The listing builds one solid part. Answer for the finished solid, in the listing's coordinates (mm). A direction names the side the tool comes from. Give positions to 0.01 mm unless a question says otherwise; leave off trailing zeros. Order: outer loops, then holes, each group sorted by start corner. A loop starts at its lowest first (then second) coordinate and runs counter-clockwise, first axis right, second up. Notation, with made-up numbers: (-32.5, 87.5) - (9.5, 87.5) arc R17 ccw to (9.5, 100.5) - close; hole circle Ø3 at (52, 78.5). An arc over 180 degrees is marked (long way). Use CSV: the item, a comma, the result in double quotes.
```python
from build123d import *

# Parameters (mm, degrees)
F0_R            = 100
F1_DEPTH        = 22
F2_R            = 3
F3_DEPTH        = 160
F3_COPIES_COUNT = 8
F4_R            = 15
F5_DEPTH        = 23
F6_R            = 5
F7_DEPTH        = 150


# Not quite as in the source:
# - a pattern or mirror of a feature is missing from the dataset's text; its kind, count and spacing are read off the source's solid


with BuildPart() as f1:
    # F0 (on Top) → F1 (new body)
    with BuildSketch(Plane.XY):
        Circle(F0_R)
    extrude(amount=F1_DEPTH)

    # F2 (on face) → F3 (join)
    with BuildSketch(Plane.XY.offset(22)):
        with Locations((10, 0)):
            Circle(F2_R)
        with Locations((30, 0)):
            Circle(F2_R)
        with Locations((50, 0)):
            Circle(F2_R)
        with Locations((70, 0)):
            Circle(F2_R)
        with Locations((90, 0)):
            Circle(F2_R)
    f3 = extrude(amount=F3_DEPTH)

    # F3_copies: F3 ×8 about axis
    f3_copies_axis = Axis((0, 0, 0), (0, 0, 1))
    for i in range(1, F3_COPIES_COUNT):
        add(f3.rotate(f3_copies_axis, i * 360 / F3_COPIES_COUNT))

    # F4 (on face) → F5 (join)
    with BuildSketch(Plane.XY):
        Circle(F4_R)
    extrude(amount=-F5_DEPTH)

    # F6 (on face) → F7 (join)
    with BuildSketch(Plane(origin=(0, 0, -23), x_dir=(1, 0, 0), z_dir=(0, 0, -1))):
        Circle(F6_R)
    extrude(amount=F7_DEPTH)


solid = f1.part
```
Item 1: The mould has two halves that part along X. Classify faces 3 (the face through (95.38, 30.04, 10.85)), 4 (the face through (-1, 1, 22)), 5 (the face through (-1, -21, 0)): +X half, -X half, draft (parallel to the pull), parting line (faces both ways), or undercut.
Taken from the geometry:
face 3,"parting line"
face 4,"undercut"
face 5,"draft"
Item 2: The part is cut by section B-B (z = -141). Give the vertices of the cut face in (x, y), and give its area (3 significant figures).
Taken from the geometry:
outline,"circle Ø10 at (0, 0)"
area,"78.5 mm^2"
Item 3: Find the intervals of material crossed by line 1 along X through (y, z) = (-63.5, 132); line 2 along Z through (x, y) = (-13, -34); line 3 along X through (y, z) = (-30, 30.5), in increasing order.
Taken from the geometry:
line 1,"-66.64 to -60.64, 60.64 to 66.64"
line 2,"0 to 22"
line 3,"-3 to 3"
Item 4: The part is cut by section A-A (z = 17.5). Give the vertices of the cut face in (x, y).
Taken from the geometry:
outline,"circle Ø200 at (0, 0)"
Item 5: Each of these flat-tipped pins is pushed along its axis until it touches: pin 1 (24 mm diameter, centred on x = 1.5, y = -5.5, fed in from -Z); pin 2 (1.5 mm diameter, centred on x = -29.5, z = 14, fed in from -Y); pin 3 (1 mm diameter, centred on x = 76.5, y = 57, fed in from -Z); pin 4 (1.5 mm diameter, centred on y = 46, z = 39, fed in from +X). Where does it stop, or does it pass through?
Taken from the geometry:
pin 1,"z = -173"
pin 2,"y = -95.78"
pin 3,"z = 0"
pin 4,"x = 50.7"
Item 6: Which of the six approach directions +Z, -Z, +X, -X, +Y, -Y give full straight-line access (tool end or side, diameter ignored) to faces 1 (the face through (-4, 4, -23)), 2 (the face through (0, 0, -173))?
Taken from the geometry:
face 1,"-Z"
face 2,"-Z, +X, -X, +Y, -Y"
